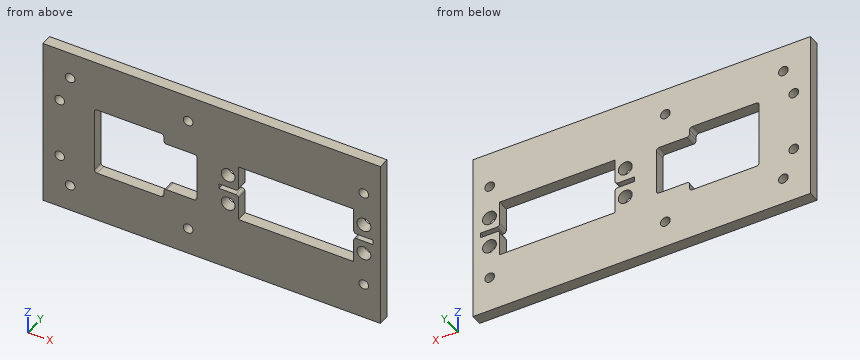
from build123d import *

# Parameters (mm, degrees)
SKETCH1_W           = 121.5
SKETCH1_H           = 62
SKETCH1_W_2         = 25
SKETCH1_H_2         = 25
BOSS_EXTRUDE1_DEPTH = 4
SKETCH2_R           = 2.5
CUT_EXTRUDE1_DEPTH  = 5
SKETCH3_R           = 1.75
CUT_EXTRUDE2_DEPTH  = 5
SKETCH4_W           = 12
SKETCH4_H           = 18
CUT_EXTRUDE3_DEPTH  = 5
FILLET1_R           = 1


with BuildPart() as part:
    # Sketch1 → Boss-Extrude1 (new body)
    with BuildSketch(Plane(origin=(0, 0, 0), x_dir=(1, 0, 0), z_dir=(0, 1, 0))):
        with Locations((10.25, 0)):
            Rectangle(SKETCH1_W, SKETCH1_H)
        with Locations((-19.5, 0)):
            Rectangle(SKETCH1_W_2, SKETCH1_H_2, mode=Mode.SUBTRACT)
    extrude(amount=BOSS_EXTRUDE1_DEPTH)

    # Sketch2 → Cut-Extrude1 (cut, through all)
    with BuildSketch(Plane(origin=(0, 4, 0), x_dir=(1, 0, 0), z_dir=(0, 1, 0))):
        with Locations((16.18, 5.6)):
            Circle(SKETCH2_R)
        with Locations((16.18, -5.6)):
            Circle(SKETCH2_R)
        with Locations((65.06, -5.6)):
            Circle(SKETCH2_R)
        with Locations((65.06, 5.6)):
            Circle(SKETCH2_R)
        Polygon((19.87, -0.9), (12.87, -0.9), (12.87, 0.9), (19.87, 0.9), (19.87, 10.4), (61.37, 10.4), (61.37, 0.9), (68.37, 0.9), (68.37, -0.9), (61.37, -0.9), (61.37, -10.4), (19.87, -10.4), align=None)
    extrude(amount=-CUT_EXTRUDE1_DEPTH, mode=Mode.SUBTRACT)

    # Sketch3 → Cut-Extrude2 (cut, through all)
    with BuildSketch(Plane(origin=(0, 4, 0), x_dir=(1, 0, 0), z_dir=(0, 1, 0))):
        with Locations((-40.75, -21.25)):
            Circle(SKETCH3_R)
        with Locations((-44.5, -11)):
            Circle(SKETCH3_R)
        with Locations((1.75, -21.25)):
            Circle(SKETCH3_R)
        with Locations((1.75, 21.25)):
            Circle(SKETCH3_R)
        with Locations((65, 18)):
            Circle(SKETCH3_R)
        with Locations((65, -18)):
            Circle(SKETCH3_R)
        with Locations((-44.5, 11)):
            Circle(SKETCH3_R)
        with Locations((-40.75, 21.25)):
            Circle(SKETCH3_R)
    extrude(amount=-CUT_EXTRUDE2_DEPTH, mode=Mode.SUBTRACT)

    # Sketch4 → Cut-Extrude3 (cut, through all)
    with BuildSketch(Plane(origin=(0, 4, 0), x_dir=(1, 0, 0), z_dir=(0, 1, 0))):
        with Locations((-1, 0)):
            Rectangle(SKETCH4_W, SKETCH4_H)
    extrude(amount=-CUT_EXTRUDE3_DEPTH, mode=Mode.SUBTRACT)

    # Fillet1
    fillet1_edges = [part.edges().sort_by_distance(p)[0] for p in [
        (-7, 2, 9),
        (-7, 2, -9),
        (5, 2, -9),
        (5, 2, 9),
        (-32, 2, -12.5),
        (-32, 2, 12.5),
        (-7, 2, 12.5),
        (-7, 2, -12.5),
        (19.87, 2, -0.9),
        (61.37, 2, -0.9),
        (61.37, 2, 0.9),
        (19.87, 2, 0.9),
    ]]
    fillet(fillet1_edges, radius=FILLET1_R)


solid = part.part
Geometry check sheet. Reference: the model listing, model coordinates, mm. Coordinates: 2 decimals unless noted, no trailing zeros. Write each loop counter-clockwise with the first axis right and the second up, starting at its lowest first coordinate (ties: lowest second). Pieces come first, ordered by that corner, then holes. Notation, with made-up numbers: (67, 4.5) -> (125, 4.5) arc R26 cw to (125, 32.5) -> close; hole circle Ø10 at (61.25, 79). An arc over 180 degrees is marked (long way). One line per question, with ' | ' between items.
1. Thickness scan on probe 1 along X at (y, z) = (1.95, 21.25); probe 2 along Z at (x, y) = (-40.75, 1.7); probe 3 along X at (y, z) = (1.8, -11). Record the ranges inside material, lowest first. Write a range as from..to.
Answers:
probe 1: x = -50.5..-42.5, -39..0, 3.5..71 | probe 2: z = -31..-23, -19.5..19.5, 23..31 | probe 3: x = -50.5..-46.25, -42.75..-32, -7..71
2. Cross-section at B-B on x = 16.18. Record the cut outline in (y, z).
Answers:
outline: (0, -31) -> (4, -31) -> (4, -8.1) -> (0, -8.1) -> close; (0, -3.1) -> (4, -3.1) -> (4, -0.9) -> (0, -0.9) -> close; (0, 0.9) -> (4, 0.9) -> (4, 3.1) -> (0, 3.1) -> close; (0, 8.1) -> (4, 8.1) -> (4, 31) -> (0, 31) -> close
3. Cross-section at D-D on x = -3.5. Record the cut outline in (y, z).
Answers:
outline: (0, -31) -> (4, -31) -> (4, -9) -> (0, -9) -> close; (0, 9) -> (4, 9) -> (4, 31) -> (0, 31) -> close
4. Cross-section at A-A on z = -21.25. Record the cut outline in (x, y).
Answers:
outline: (-50.5, 0) -> (-42.5, 0) -> (-42.5, 4) -> (-50.5, 4) -> close; (-39, 0) -> (0, 0) -> (0, 4) -> (-39, 4) -> close; (3.5, 0) -> (71, 0) -> (71, 4) -> (3.5, 4) -> close
5. Cross-section at C-C on z = -5.6. Record the cut outline in (x, y), and give its area (3 significant figures).
Answers:
outline: (-50.5, 0) -> (-32, 0) -> (-32, 4) -> (-50.5, 4) -> close; (5, 0) -> (13.68, 0) -> (13.68, 4) -> (5, 4) -> close; (18.68, 0) -> (19.87, 0) -> (19.87, 4) -> (18.68, 4) -> close; (61.37, 0) -> (62.56, 0) -> (62.56, 4) -> (61.37, 4) -> close; (67.56, 0) -> (71, 0) -> (71, 4) -> (67.56, 4) -> close | area: 132 mm²
6. Depth check by flat-ended pin: pin 1 Ø3 at (x, z) = (65.06, 5.6) entering from -Y. Enter the tip coordinate at first touch or a pass-through.
Answers:
pin 1: passes through
